CAD build for the part. Positions are in the model's coordinates, mm. A direction names the side the tool comes from. Round coordinates to 2 decimals unless told otherwise and drop trailing zeros. Write each loop counter-clockwise with the first axis right and the second up, starting at its lowest first coordinate (ties: lowest second). Pieces come first, ordered by that corner, then holes. Notation, with made-up numbers: (36, -17) - (88, -17) arc R30 cw to (88, 19) - close; hole circle Ø8 at (47.25, 3.25). An arc over 180 degrees is marked (long way). Put each result on its own line as item: value. Start each with the question number.
Item 1: Drill centre lines: line 1 (Y direction, x = 0.75, z = 5.25); line 2 (Y direction, x = 1, z = 3.25); line 3 (X direction, y = -1.75, z = -1.25). Where is each one in solid material? Low to high. Write a range as from..to.
Item 2: Mould opens along X. For faces 6 (the flat face through (0, -2, 2)), 7 (the flat face through (5.081, -4.93, 2.876)), 8 (the flat face through (-4.76, -4.93, 3.79)) say: released by +X, released by -X, zero draft, split by the parting line, or undercut.
Item 3: Cut at D-D (x = -3). Give the cut face in (y, z).
Item 4: 3-axis set-ups, long thin cutter, end or side, ignore diameter. For faces 1 (the flat face through (4.7, -10, 3.4)), 2 (the flat face through (1, -1, 0)), 3 (the flat face through (-4.77, -4.93, -0.61)), 4 (the flat face through (-5.08, -4.93, 0.3)), 5 (the flat face through (5.09, -4.93, 0.28)): which of +Z, -Z, +X, -X, +Y, -Y reach the whole face in a straight line?
Item 5: Cut at C-C (z = 4.5). Give the cut face in (x, y).
Item 6: Pin check, flat tips, straight feed: pin 1 Ø1 at (x, z) = (2.5, -0.5) entering from -Y; pin 2 Ø2 at (y, z) = (-5, -2) entering from +X; pin 3 Ø1.5 at (y, z) = (-3.5, 4) entering from -X; pin 4 Ø3 at (x, y) = (-3.5, -6) entering from -Z. Stop position of each tip, or through.
Item 7: Cut at A-A (y = -3.25). Give the cut face in (x, z).
Item 8: Cut at B-B (x = 0). Give the cut face in (y, z).
```python
from build123d import *

# Parameters (mm, degrees)
F1_DEPTH = 2
F2_DEPTH = 10
F3_R     = 3.2545252872
F4_DEPTH = 1
F5_R     = 1.6545252872
F6_DEPTH = 1


with BuildPart() as f1:
    # F0 (on Front) → F1 (new body)
    with BuildSketch(Plane.XZ):
        with BuildLine():
            ThreePointArc((4.6885970941, 0.8556488446), (4.7312339405, 1.2208070974), (4.7454747128, 1.588170202))
            ThreePointArc((4.7454747128, 1.588170202), (4.7312339405, 1.9555333066), (4.6885970941, 2.3206915594))
            Line((4.6885970941, 2.3206915594), (3.5662952021, 2.8547403321))
            Line((3.5662952021, 2.8547403321), (4.1003439748, 3.9770422242))
            ThreePointArc((4.1003439748, 3.9770422242), (0, 6.3336449148), (-4.1003439748, 3.9770422242))
            Line((-4.1003439748, 3.9770422242), (-3.5662952021, 2.8547403321))
            Line((-3.5662952021, 2.8547403321), (-4.6885970941, 2.3206915594))
            ThreePointArc((-4.6885970941, 2.3206915594), (-4.7454747128, 1.588170202), (-4.6885970941, 0.8556488446))
            Line((-4.6885970941, 0.8556488446), (-3.5662952021, 0.3216000719))
            Line((-3.5662952021, 0.3216000719), (-4.1003439748, -0.8007018202))
            ThreePointArc((-4.1003439748, -0.8007018202), (0, -3.1573045108), (4.1003439748, -0.8007018202))
            Line((4.1003439748, -0.8007018202), (3.5662952021, 0.3216000719))
            Line((3.5662952021, 0.3216000719), (4.6885970941, 0.8556488446))
        make_face()
        with BuildLine():
            Line((-3.5662952021, 2.8547403321), (-4.1003439748, 3.9770422242))
            ThreePointArc((-4.1003439748, 3.9770422242), (-4.4718279998, 3.176340404), (-4.6885970941, 2.3206915594))
            Line((-4.6885970941, 2.3206915594), (-3.5662952021, 2.8547403321))
        make_face()
        with BuildLine():
            ThreePointArc((-4.6885970941, 2.3206915594), (-4.4718279998, 3.176340404), (-4.1003439748, 3.9770422242))
            Line((-4.1003439748, 3.9770422242), (-4.1502279279, 4.0818732017))
            Line((-4.1502279279, 4.0818732017), (-5.3773607975, 3.4979404759))
            Line((-5.3773607975, 3.4979404759), (-4.7934280717, 2.2708076063))
            Line((-4.7934280717, 2.2708076063), (-4.6885970941, 2.3206915594))
        make_face()
        with BuildLine():
            ThreePointArc((-4.6885970941, 0.8556488446), (-4.4718279998, 0), (-4.1003439748, -0.8007018202))
            Line((-4.1003439748, -0.8007018202), (-3.5662952021, 0.3216000719))
            Line((-3.5662952021, 0.3216000719), (-4.6885970941, 0.8556488446))
        make_face()
        with BuildLine():
            Line((-4.1502279279, -0.9055327977), (-4.1003439748, -0.8007018202))
            ThreePointArc((-4.1003439748, -0.8007018202), (-4.4718279998, 0), (-4.6885970941, 0.8556488446))
            Line((-4.6885970941, 0.8556488446), (-4.7934280717, 0.9055327977))
            Line((-4.7934280717, 0.9055327977), (-5.3773607975, -0.3216000719))
            Line((-5.3773607975, -0.3216000719), (-4.1502279279, -0.9055327977))
        make_face()
        with BuildLine():
            Line((4.7934280717, 0.9055327977), (4.6885970941, 0.8556488446))
            ThreePointArc((4.6885970941, 0.8556488446), (4.4718279998, 0), (4.1003439748, -0.8007018202))
            Line((4.1003439748, -0.8007018202), (4.1502279279, -0.9055327977))
            Line((4.1502279279, -0.9055327977), (5.3773607975, -0.3216000719))
            Line((5.3773607975, -0.3216000719), (4.7934280717, 0.9055327977))
        make_face()
        with BuildLine():
            ThreePointArc((4.1003439748, -0.8007018202), (4.4718279998, 0), (4.6885970941, 0.8556488446))
            Line((4.6885970941, 0.8556488446), (3.5662952021, 0.3216000719))
            Line((3.5662952021, 0.3216000719), (4.1003439748, -0.8007018202))
        make_face()
        with BuildLine():
            Line((3.5662952021, 2.8547403321), (4.6885970941, 2.3206915594))
            ThreePointArc((4.6885970941, 2.3206915594), (4.4718279998, 3.176340404), (4.1003439748, 3.9770422242))
            Line((4.1003439748, 3.9770422242), (3.5662952021, 2.8547403321))
        make_face()
        with BuildLine():
            ThreePointArc((4.1003439748, 3.9770422242), (4.4718279998, 3.176340404), (4.6885970941, 2.3206915594))
            Line((4.6885970941, 2.3206915594), (4.7934280717, 2.2708076063))
            Line((4.7934280717, 2.2708076063), (5.3773607975, 3.4979404759))
            Line((5.3773607975, 3.4979404759), (4.1502279279, 4.0818732017))
            Line((4.1502279279, 4.0818732017), (4.1003439748, 3.9770422242))
        make_face()
    extrude(amount=F1_DEPTH)

    # F0 (on Front) → F2 (join)
    with BuildSketch(Plane.XZ):
        with BuildLine():
            ThreePointArc((-4.6885970941, 2.3206915594), (-4.4718279998, 3.176340404), (-4.1003439748, 3.9770422242))
            Line((-4.1003439748, 3.9770422242), (-4.1502279279, 4.0818732017))
            Line((-4.1502279279, 4.0818732017), (-5.3773607975, 3.4979404759))
            Line((-5.3773607975, 3.4979404759), (-4.7934280717, 2.2708076063))
            Line((-4.7934280717, 2.2708076063), (-4.6885970941, 2.3206915594))
        make_face()
        with BuildLine():
            Line((-4.1502279279, -0.9055327977), (-4.1003439748, -0.8007018202))
            ThreePointArc((-4.1003439748, -0.8007018202), (-4.4718279998, 0), (-4.6885970941, 0.8556488446))
            Line((-4.6885970941, 0.8556488446), (-4.7934280717, 0.9055327977))
            Line((-4.7934280717, 0.9055327977), (-5.3773607975, -0.3216000719))
            Line((-5.3773607975, -0.3216000719), (-4.1502279279, -0.9055327977))
        make_face()
        with BuildLine():
            Line((4.7934280717, 0.9055327977), (4.6885970941, 0.8556488446))
            ThreePointArc((4.6885970941, 0.8556488446), (4.4718279998, 0), (4.1003439748, -0.8007018202))
            Line((4.1003439748, -0.8007018202), (4.1502279279, -0.9055327977))
            Line((4.1502279279, -0.9055327977), (5.3773607975, -0.3216000719))
            Line((5.3773607975, -0.3216000719), (4.7934280717, 0.9055327977))
        make_face()
        with BuildLine():
            ThreePointArc((4.1003439748, 3.9770422242), (4.4718279998, 3.176340404), (4.6885970941, 2.3206915594))
            Line((4.6885970941, 2.3206915594), (4.7934280717, 2.2708076063))
            Line((4.7934280717, 2.2708076063), (5.3773607975, 3.4979404759))
            Line((5.3773607975, 3.4979404759), (4.1502279279, 4.0818732017))
            Line((4.1502279279, 4.0818732017), (4.1003439748, 3.9770422242))
        make_face()
    extrude(amount=F2_DEPTH)

    # F3 (on face) → F4 (cut)
    with BuildSketch(Plane.XZ.offset(2)):
        with Locations((0, 1.588170202)):
            Circle(F3_R)
    extrude(amount=-F4_DEPTH, mode=Mode.SUBTRACT)

    # F5 (on face) → F6 (join)
    with BuildSketch(Plane.XZ.offset(1)):
        with Locations((0, 1.588170202)):
            Circle(F5_R)
    extrude(amount=F6_DEPTH)


solid = f1.part
```
Output values:
1. line 1: -2..0
1. line 2: -1..0
1. line 3: -3.8..-1.59, 1.59..3.8
2. face 6: undercut
2. face 7: released by +X
2. face 8: released by -X
3. outline: (-2, -2.09) - (0, -2.09) - (0, 5.27) - (-2, 5.27) - (-2, 2.85) - (-1, 2.85) - (-1, 0.33) - (-2, 0.33) - close
4. face 1: +Z, -Z, +X, -X, -Y
4. face 2: -Y
4. face 3: -Z, -X, +Y, -Y
4. face 4: -X, +Y, -Y
4. face 5: +X, +Y, -Y
5. outline: (-3.75, -2) - (-1.45, -2) - (-1.45, -1) - (1.45, -1) - (1.45, -2) - (3.75, -2) - (3.75, 0) - (-3.75, 0) - close
6. pin 1: y = -2
6. pin 2: through
6. pin 3: x = -5.38
6. pin 4: z = -0.91
7. outline: (-5.38, -0.32) - (-4.15, -0.91) - (-4.1, -0.8) arc R4.75 cw to (-4.69, 0.86) - (-4.79, 0.91) - close; (-5.38, 3.5) - (-4.79, 2.27) - (-4.69, 2.32) arc R4.75 cw to (-4.1, 3.98) - (-4.15, 4.08) - close; (4.1, -0.8) - (4.15, -0.91) - (5.38, -0.32) - (4.79, 0.91) - (4.69, 0.86) arc R4.75 cw to start; (4.1, 3.98) arc R4.75 cw to (4.69, 2.32) - (4.79, 2.27) - (5.38, 3.5) - (4.15, 4.08) - close
8. outline: (-2, -3.16) - (0, -3.16) - (0, 6.33) - (-2, 6.33) - (-2, 4.84) - (-1, 4.84) - (-1, 3.24) - (-2, 3.24) - (-2, -0.07) - (-1, -0.07) - (-1, -1.67) - (-2, -1.67) - close
